Work out the finished part from the listing and answer in its coordinate system (mm). A direction names the side the tool comes from. Round coordinates to 2 decimals unless told otherwise and drop trailing zeros. Order: outer loops, then holes, each group sorted by start corner. A loop starts at its lowest first (then second) coordinate and runs counter-clockwise, first axis right, second up. Notation, with made-up numbers: M -29,16.5 L 2,16.5 A27 cw 2,55.5 Z; hole C 56.5,0 d5. An arc over 180 degrees is marked long. Return JSON: item names as keys, results as strings.
from build123d import *

# Parameters (mm, degrees)
EXTRUDE_2_DEPTH     = 33.8
SKETCH_2_W          = 63
SKETCH_2_H          = 27.8
CUT_EXTRUDE_2_DEPTH = 73.190304058
SKETCH_4_W          = 15
SKETCH_4_H          = 13.9
EXTRUDE_4_DEPTH     = 10
FILLET_1_R          = 5
FILLET_2_R          = 5
FILLET_3_R          = 2.5
SKETCH_5_R          = 2.5
CUT_EXTRUDE_3_DEPTH = 72.668961204
SKETCH_6_R          = 1
CUT_EXTRUDE_4_DEPTH = 72.668961204
CHAMFER_2_SIZE      = 0.5


with BuildPart() as part:
    # Sketch 1 → Extrude 2 (new body)
    with BuildSketch(Plane(origin=(0, 0, 0), x_dir=(1, 0, 0), z_dir=(0, 1, 0))):
        with BuildLine():
            Line((-5, 0), (0, 0))
            Line((0, 0), (0, 58))
            Line((0, 58), (0, 63))
            ThreePointArc((0, 63), (-3.535533906, 61.535533906), (-5, 58))
            Line((-5, 58), (-5, 0))
        make_face()
        with BuildLine():
            Line((0, 58), (0, 0))
            Line((0, 0), (5, 0))
            Line((5, 0), (5, 58))
            ThreePointArc((5, 58), (3.535533906, 61.535533906), (0, 63))
            Line((0, 63), (0, 58))
        make_face()
        with BuildLine():
            ThreePointArc((-5, 58), (-3.535533906, 61.535533906), (0, 63))
            Line((0, 63), (-5, 63))
            Line((-5, 63), (-5, 58))
        make_face()
        with BuildLine():
            Line((5, 63), (0, 63))
            ThreePointArc((0, 63), (3.535533906, 61.535533906), (5, 58))
            Line((5, 58), (5, 63))
        make_face()
    extrude(amount=EXTRUDE_2_DEPTH)

    # Sketch 2 → Cut-Extrude 2 (cut, through all)
    with BuildSketch(Plane.ZY.offset(5)):
        with Locations((-31.5, 16.9)):
            Rectangle(SKETCH_2_W, SKETCH_2_H)
    extrude(amount=-CUT_EXTRUDE_2_DEPTH, mode=Mode.SUBTRACT)


with BuildPart() as cut_extrude_2_piece_1:
    # of the separate pieces the step leaves, piece 1, a body of its own (cut_extrude_2_pieces)
    add(part.part.solids().sort_by_distance((-5, 30.8, 0))[0])



with BuildPart() as cut_extrude_2_piece_2:
    # of the separate pieces the step leaves, piece 2, a body of its own (cut_extrude_2_pieces)
    add(part.part.solids().sort_by_distance((-5, 0, 0))[0])


with BuildPart() as cut_extrude_2_piece_1_1:
    add(cut_extrude_2_piece_1.part)

    add(cut_extrude_2_piece_2.part)  # Extrude 4 merges Cut-Extrude 2 piece 2
    # Sketch 4 → Extrude 4 (add)
    with BuildSketch(Plane.ZY.offset(5)):
        Polygon((0, 3), (0, 0), (15, 3), align=None)
        with Locations((7.5, 9.95)):
            Rectangle(SKETCH_4_W, SKETCH_4_H)
        with Locations((7.5, 23.85)):
            Rectangle(SKETCH_4_W, SKETCH_4_H)
        Polygon((0, 33.8), (0, 30.8), (15, 30.8), align=None)
    extrude(amount=-EXTRUDE_4_DEPTH)

    # Fillet 1
    fillet_1_edges = [cut_extrude_2_piece_1_1.edges().sort_by_distance(p)[0] for p in [
        (5, 1.5, -63),
        (-5, 1.5, -63),
        (5, 32.3, -63),
        (-5, 32.3, -63),
    ]]
    fillet(fillet_1_edges, radius=FILLET_1_R - 0.0001)  # a hair under: the kernel refuses the full size

    # Fillet 2
    fillet_2_edges = [cut_extrude_2_piece_1_1.edges().sort_by_distance(p)[0] for p in [
        (0, 30.8, 0),
        (0, 3, 0),
    ]]
    fillet(fillet_2_edges, radius=FILLET_2_R)

    # Fillet 3
    fillet_3_edges = [cut_extrude_2_piece_1_1.edges().sort_by_distance(p)[0] for p in [
        (0, 30.8, 15),
        (0, 3, 15),
    ]]
    fillet(fillet_3_edges, radius=FILLET_3_R)

    # Sketch 5 → Cut-Extrude 3 (cut, through all)
    with BuildSketch(Plane(origin=(0, 33.8, 0), x_dir=(1, 0, 0), z_dir=(0, 1, 0))):
        with Locations(Location((0, 58, 0), (0, 0, 270))):
            Circle(SKETCH_5_R)
    extrude(amount=-CUT_EXTRUDE_3_DEPTH, mode=Mode.SUBTRACT)

    # Sketch 6 → Cut-Extrude 4 (cut, through all)
    with BuildSketch(Plane(origin=(0, 0, 0), x_dir=(-1, 0, 0), z_dir=(0, 0, -1))):
        with Locations((0, 16.9)):
            Circle(SKETCH_6_R)
    extrude(amount=-CUT_EXTRUDE_4_DEPTH, mode=Mode.SUBTRACT)

    # Chamfer 2
    chamfer_2_edges = [cut_extrude_2_piece_1_1.edges().sort_by_distance(p)[0] for p in [
        (-5, 1.299029034, 6.495145169),
        (5, 32.500970966, 6.495145169),
        (5, 33.8, -29.00005),
        (5, 0, -29.00005),
        (-5, 0, -29.00005),
        (-3.535563195, 0, -61.535563195),
        (3.535563195, 0, -61.535563195),
        (5, 30.8, -31.50005),
        (5, 3, -31.50005),
        (-5, 3, -31.50005),
        (-3.535563195, 3, -61.535563195),
        (3.535563195, 3, -61.535563195),
        (-5, 30.8, -31.50005),
        (-5, 33.8, -29.00005),
        (-3.535563195, 30.8, -61.535563195),
        (3.535563195, 30.8, -61.535563195),
        (-3.535563195, 33.8, -61.535563195),
        (3.535563195, 33.8, -61.535563195),
        (-5, 16.9, 0),
        (5, 16.9, 0),
        (-5, 29.335533906, -1.464466094),
        (5, 29.335533906, -1.464466094),
        (-5, 4.464466094, -1.464466094),
        (5, 4.464466094, -1.464466094),
        (5, 16.9, 15),
        (-5, 16.9, 15),
        (-5, 32.500970966, 6.495145169),
        (-5, 3.464537493, 14.433355353),
        (-5, 30.335462507, 14.433355353),
        (5, 1.299029034, 6.495145169),
        (5, 3.464537493, 14.433355353),
        (5, 30.335462507, 14.433355353),
    ]]
    chamfer(chamfer_2_edges, length=CHAMFER_2_SIZE)


solid = cut_extrude_2_piece_1_1.part
Item 1: Find section C-C (x = 1.75). State how many separate pieces and enclosed holes the cut face has, plus the area to 3 significant figures.
Output:
{"separate pieces": "3", "enclosed holes": "0", "area": "825 mm^2"}
Item 2: Consider line 1 along Y through (x, z) = (2.5, -15); line 2 along X through (y, z) = (1, -58); line 3 along Z through (x, y) = (0.5, 13). Determine where each line is inside the solid, lowest interval first. Write a range as [from, to].
Output:
{"line 1": "y = [0, 3], [30.8, 33.8]", "line 2": "x = [-5, -2.5], [2.5, 5]", "line 3": "z = [0, 15]"}
Item 3: The mould has two halves that part along Y. Classify faces 1 (the conical face through (3.314, 2.865, -61.242)), 2 (the cylindrical face through (4, 2, -61)), 3 (the conical face through (4.858, 3.675, 14.144)), 4 (the conical face through (-3.314, 30.935, -61.242)): pulls with the +Y half, pulls with the -Y half, needs draft (parallel to the pull), parting line crosses it, or undercut.
Output:
{"face 1": "undercut", "face 2": "needs draft", "face 3": "pulls with the -Y half", "face 4": "undercut"}
Item 4: Which of the six approach directions +Z, -Z, +X, -X, +Y, -Y give full straight-line access (tool end or side, diameter ignored) to faces 5 (the conical face through (-3.242, 0.135, -61.314)), 6 (the flat face through (0, 15, 0)), 7 (the conical face through (-4.635, 29.391, -1.329))?
Output:
{"face 5": "-Z, -X, -Y", "face 6": "-Z, +X, -X", "face 7": "-Z, -X"}
Item 5: Find section A-A (z = -8). Determine the outline of the cut face in (x, y).
Output:
{"outline": "M -5,0.5 L -4.5,0 L 4.5,0 L 5,0.5 L 5,2.5 L 4.5,3 L -4.5,3 L -5,2.5 Z; M -5,31.3 L -4.5,30.8 L 4.5,30.8 L 5,31.3 L 5,33.3 L 4.5,33.8 L -4.5,33.8 L -5,33.3 Z"}
Item 6: Find section B-B (y = 16.9). Determine the outline of the cut face in (x, z), plus the area to 4 significant figures.
Output:
{"outline": "M -5,0.5 L -4.5,0 L -1,0 L -1,15 L -4.5,15 L -5,14.5 Z; M 1,0 L 4.5,0 L 5,0.5 L 5,14.5 L 4.5,15 L 1,15 Z", "area": "119.5 mm^2"}
Item 7: This flat-tipped pin is pushed along its axis until it touches: pin 1 (2.5 mm diameter, centred on x = 2, y = 21, fed in from -Z). Where does it stop, or does it pass through?
Output:
{"pin 1": "stops at z = 0"}
